```python
from build123d import *

# Parameters (mm, degrees)
F0_W     = 80
F0_H     = 202
F1_DEPTH = 3
F2_W     = 41.942806
F2_H     = 44
F2_W_2   = 43.622092
F3_DEPTH = 25


with BuildPart() as f1:
    # F0 (on Front) → F1 (new body)
    with BuildSketch(Plane.XZ):
        with Locations((-19.744222, 27.878283)):
            Rectangle(F0_W, F0_H)
    extrude(amount=F1_DEPTH)

    # F2 (on face) → F3 (cut)
    with BuildSketch(Plane.XZ.offset(3)):
        with Locations((-34.772819, 52.878283)):
            Rectangle(F2_W, F2_H)
        with Locations((-5.555268, 102.878283)):
            Rectangle(F2_W_2, F2_H)
        Polygon((16.255778, -25.121717), (-41.454826, -25.121717), (-41.454826, -42.175964), (-41.454826, -69.121717), (16.255778, -69.121717), align=None)
    extrude(amount=-F3_DEPTH, mode=Mode.SUBTRACT)


solid = f1.part
```
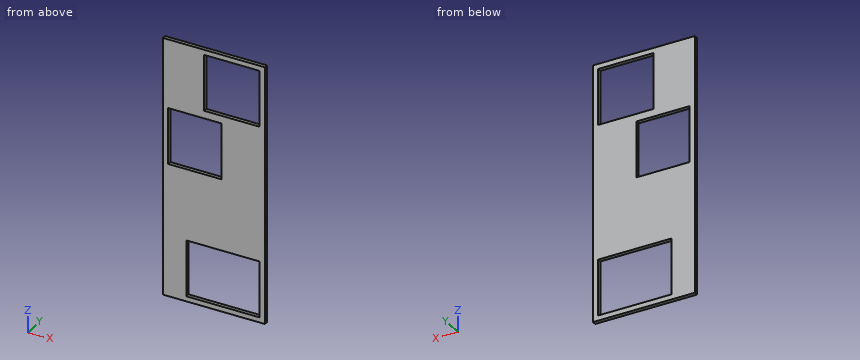
Can you work these out from the model? Positions are in its coordinate system, mm. Round coordinates to 2 decimals unless told otherwise and drop trailing zeros. Loops run counter-clockwise (first coordinate to the right, second up) from the corner with the lowest first, then second, coordinate; pieces in that order, holes last. Notation, with made-up numbers: M 56.5,-21 L 91.5,-21 A19 cw 91.5,0 Z; hole C -29,65 d10. An arc over 180 degrees is marked long. Write item = value, one per line. Start each with the question number.
(1) Suppose I cut it at D-D on y = -0.9. Write out the boundary of the cut face in (x, z).
(2) Suppose I cut it at A-A on z = -34. Write out the boundary of the cut face in (x, y).
(3) Suppose I cut it at C-C on x = -49.5. Write out the boundary of the cut face in (y, z), plus the area to 3 significant figures.
(4) Suppose I cut it at B-B on x = -35.5. Write out the boundary of the cut face in (y, z).
(5) I need wall thicknesses on line 1 along Z through (x, y) = (8, -0.6); line 2 along Z through (x, y) = (-40.5, -1.6); line 3 along Z through (x, y) = (-20.5, -1.15). Which ranges of each line are inside material? Lowest first, please.
Answer block:
q1.outline = M -59.74,-73.12 L 20.26,-73.12 L 20.26,128.88 L -59.74,128.88 Z; hole M -55.74,30.88 L -13.8,30.88 L -13.8,74.88 L -55.74,74.88 Z; hole M -41.45,-69.12 L 16.26,-69.12 L 16.26,-25.12 L -41.45,-25.12 Z; hole M -27.37,80.88 L 16.26,80.88 L 16.26,124.88 L -27.37,124.88 Z
q2.outline = M -59.74,-3 L -41.45,-3 L -41.45,0 L -59.74,0 Z; M 16.26,-3 L 20.26,-3 L 20.26,0 L 16.26,0 Z
q3.outline = M -3,-73.12 L 0,-73.12 L 0,30.88 L -3,30.88 Z; M -3,74.88 L 0,74.88 L 0,128.88 L -3,128.88 Z
q3.area = 474 mm²
q4.outline = M -3,-73.12 L 0,-73.12 L 0,-69.12 L -3,-69.12 Z; M -3,-25.12 L 0,-25.12 L 0,30.88 L -3,30.88 Z; M -3,74.88 L 0,74.88 L 0,128.88 L -3,128.88 Z
q5.line_1 = -73.12 to -69.12, -25.12 to 80.88, 124.88 to 128.88
q5.line_2 = -73.12 to -69.12, -25.12 to 30.88, 74.88 to 128.88
q5.line_3 = -73.12 to -69.12, -25.12 to 30.88, 74.88 to 80.88, 124.88 to 128.88
